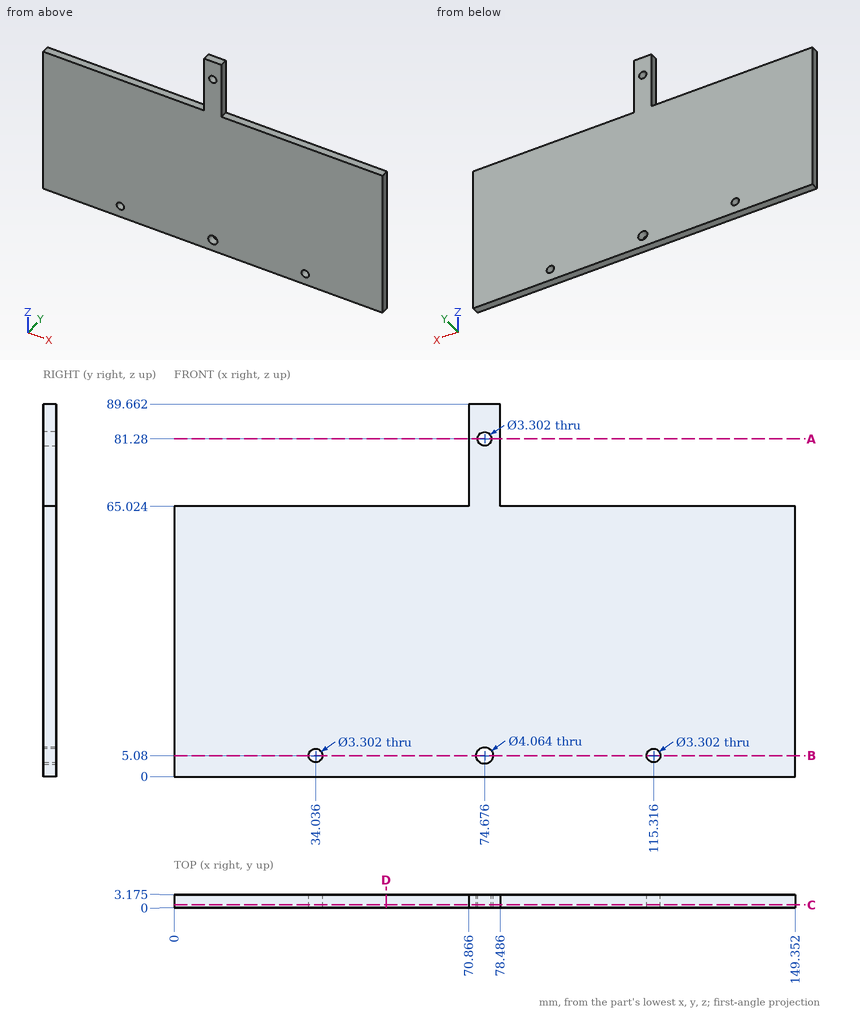
Input: dimensioned drawing with shaded views. Units: mm. Origin: part minimum x, y, z. Give positions to 0.01 mm unless a question says otherwise; leave off trailing zeros. Write each loop counter-clockwise with the first axis right and the second up, starting at its lowest first coordinate (ties: lowest second). Pieces come first, ordered by that corner, then holes. Notation, with made-up numbers: (4.25, -2.5) -> (61.25, -2.5) arc R26 cw to (61.25, 34.5) -> close; hole circle Ø1 at (55, 57). An arc over 180 degrees is marked (long way). Return JSON: item names as keys, results as strings. Group by question number.
1. Section C-C, the plane y = 0.75. Output: boundary loops of the cut face in (x, z).
2. Section A-A, the plane z = 81.28. Output: boundary loops of the cut face in (x, y) (3 decimals).
3. Material intervals for line 1 (X direction, y = 1.95, z = 5.08) (3 decimals); line 2 (X direction, y = 1.7, z = 81.28) (3 decimals); line 3 (Z direction, x = 92.5, y = 2.15), sorted ascending. Write a range as from..to.
4. Pin query (flat end, axial travel): pin 1 Ø1.6 at (y, z) = (1, 73) entering from -X; pin 2 Ø1 at (x, y) = (22, 1) entering from +Z. Return the tip coordinate at first contact, or that it passes through.
5. Section B-B, the plane z = 5.08. Output: boundary loops of the cut face in (x, y) (3 decimals), then the cut area to 3 significant figures.
6. Section D-D, the plane x = 51. Output: boundary loops of the cut face in (y, z) (3 decimals), then the cut area to 3 significant figures.
Determined:
{
 "1": {"outline": "(0, 0) -> (149.35, 0) -> (149.35, 65.02) -> (78.49, 65.02) -> (78.49, 89.66) -> (70.87, 89.66) -> (70.87, 65.02) -> (0, 65.02) -> close; hole circle Ø3.3 at (34.04, 5.08); hole circle Ø4.06 at (74.68, 5.08); hole circle Ø3.3 at (74.68, 81.28); hole circle Ø3.3 at (115.32, 5.08)"},
 "2": {"outline": "(70.866, 0) -> (73.025, 0) -> (73.025, 3.175) -> (70.866, 3.175) -> close; (76.327, 0) -> (78.486, 0) -> (78.486, 3.175) -> (76.327, 3.175) -> close"},
 "3": {"line 1": "x = 0..32.385, 35.687..72.644, 76.708..113.665, 116.967..149.352", "line 2": "x = 70.866..73.025, 76.327..78.486", "line 3": "z = 0..65.02"},
 "4": {"pin 1": "stops at x = 70.87", "pin 2": "stops at z = 65.02"},
 "5": {"outline": "(0, 0) -> (32.385, 0) -> (32.385, 3.175) -> (0, 3.175) -> close; (35.687, 0) -> (72.644, 0) -> (72.644, 3.175) -> (35.687, 3.175) -> close; (76.708, 0) -> (113.665, 0) -> (113.665, 3.175) -> (76.708, 3.175) -> close; (116.967, 0) -> (149.352, 0) -> (149.352, 3.175) -> (116.967, 3.175) -> close", "area": "440 mm2"},
 "6": {"outline": "(0, 0) -> (3.175, 0) -> (3.175, 65.024) -> (0, 65.024) -> close", "area": "206 mm2"}
}
